Build history of the part. All positions in model axes, mm. A direction names the side the tool comes from. Round coordinates to 2 decimals unless told otherwise and drop trailing zeros. Order: outer loops, then holes, each group sorted by start corner. A loop starts at its lowest first (then second) coordinate and runs counter-clockwise, first axis right, second up. Notation, with made-up numbers: M 24.5,-10 L 36.5,-10 A26 cw 36.5,5 Z; hole C 85,32.25 d9. An arc over 180 degrees is marked long. One line per item, written item: value. Start each with the question number.
Item 1: Band-saw the part on D-D, the plane x = 11.75. Write the cut outline in (y, z).
Item 2: Tool access for faces 1 (the flat face through (12, 3.5, 2)), 2 (the flat face through (0, 3, 2)): list every direction of +Z, -Z, +X, -X, +Y, -Y with a clear straight run to the whole face (end or side of a thin tool).
Item 3: Band-saw the part on A-A, the plane x = 3. Write the cut outline in (y, z).
Item 4: Band-saw the part on B-B, the plane y = 3.3. Write the cut outline in (x, z).
Item 5: Probe L1, parallel to X at y = 2.65, z = 4.7; L2, parallel to X at y = 1.4, z = 4.6; L3, parallel to Y at x = 7.5, z = 2.5. List the from-to ranges inside material, lowest first.
Item 6: Two-plate mould, pull along X, no slides. Class faces 3 (the flat face through (8, 5, 2)), 4 (the flat face through (15, 2, 2)), 5 (the flat face through (12, 1.5, 2)): +X half, -X half, draft (parallel to the pull), parting line (faces both ways), or undercut.
Item 7: Band-saw the part on C-C, the plane z = 0.9. Write the cut outline in (x, y).
```python
from build123d import *

# Parameters (mm, degrees)
SKETCH1_W           = 2.5
SKETCH1_H           = 2.5
SKETCH1_W_2         = 2
SKETCH1_H_2         = 2
SKETCH1_W_3         = 3
SKETCH1_H_3         = 3
BOSS_EXTRUDE1_DEPTH = 5


with BuildPart() as part:
    # Sketch1 → Boss-Extrude1 (new body)
    with BuildSketch(Plane.XY):
        Polygon((0, 0), (5, 0), (15, 0), (15, 5), (5, 5), (0, 5), align=None)
        with Locations((2.5, 2.5)):
            Rectangle(SKETCH1_W, SKETCH1_H, mode=Mode.SUBTRACT)
        with Locations((12.5, 2.5)):
            Rectangle(SKETCH1_W_2, SKETCH1_H_2, mode=Mode.SUBTRACT)
        with Locations((7.5, 2.5)):
            Rectangle(SKETCH1_W_3, SKETCH1_H_3, mode=Mode.SUBTRACT)
    extrude(amount=BOSS_EXTRUDE1_DEPTH)


solid = part.part
```
Output:
1. outline: M 0,0 L 1.5,0 L 1.5,5 L 0,5 Z; M 3.5,0 L 5,0 L 5,5 L 3.5,5 Z
2. face 1: +Z, -Z
2. face 2: +Z, -Z, -X, +Y, -Y
3. outline: M 0,0 L 1.25,0 L 1.25,5 L 0,5 Z; M 3.75,0 L 5,0 L 5,5 L 3.75,5 Z
4. outline: M 0,0 L 1.25,0 L 1.25,5 L 0,5 Z; M 3.75,0 L 6,0 L 6,5 L 3.75,5 Z; M 9,0 L 11.5,0 L 11.5,5 L 9,5 Z; M 13.5,0 L 15,0 L 15,5 L 13.5,5 Z
5. L1: x = 0 to 1.25, 3.75 to 6, 9 to 11.5, 13.5 to 15
5. L2: x = 0 to 1.25, 3.75 to 6, 9 to 15
5. L3: y = 0 to 1, 4 to 5
6. face 3: draft
6. face 4: +X half
6. face 5: undercut
7. outline: M 0,0 L 15,0 L 15,5 L 0,5 Z; hole M 1.25,1.25 L 3.75,1.25 L 3.75,3.75 L 1.25,3.75 Z; hole M 6,1 L 9,1 L 9,4 L 6,4 Z; hole M 11.5,1.5 L 13.5,1.5 L 13.5,3.5 L 11.5,3.5 Z
